Job drawing, mm, ordinate dimensions from the low corner. One solid piece. A direction names the side the tool comes from. Give positions to 0.01 mm unless a question says otherwise; leave off trailing zeros. Write each loop counter-clockwise with the first axis right and the second up, starting at its lowest first coordinate (ties: lowest second). Pieces come first, ordered by that corner, then holes. Notation, with made-up numbers: (15.5, 70) - (36.5, 70) arc R13 cw to (36.5, 89) - close; hole circle Ø7 at (6, -18). An arc over 180 degrees is marked (long way). Use a Markdown table: item, result. Add a question column.
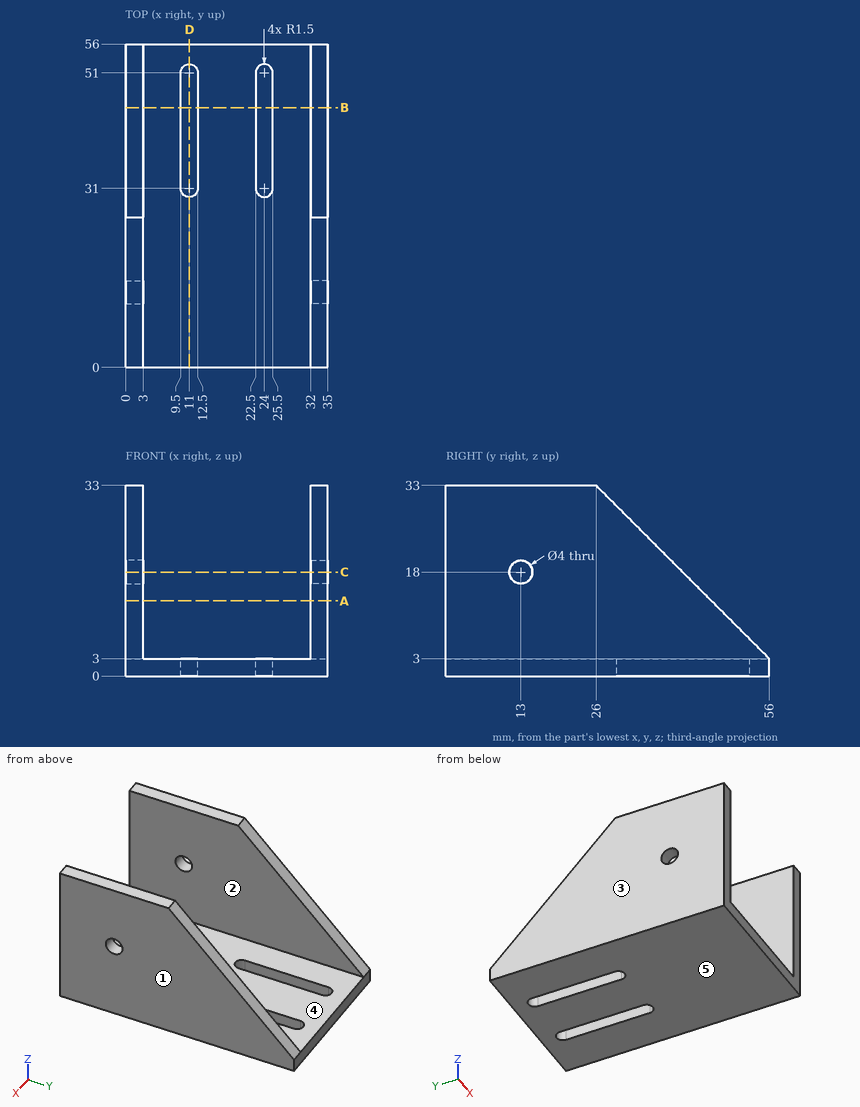
(1) Band-saw the part on C-C (z = 18). Write the cut outline in (x, y).
(2) Which spindle directions (+Z, -Z, +X, -X, +Y, -Y) get a long thin tool onto all of the face, cutting with end or side? Do the marked faces 4 and 5. Say none if no direction does.
(3) Band-saw the part on D-D (x = 11). Write the cut outline in (y, z).
(4) Flat gauge pin, fed straight in: pin 1 (12 mm diameter, centred on x = 27, z = 16, fed in from +Y). Where does the tip first touch, or does it go through?
(5) Two-plate mould, pull along X, no slides. Class the marked faces 1, 2 and 3: +X half, -X half, draft (parallel to the pull), parting line (faces both ways), or undercut.
(6) Band-saw the part on A-A (z = 13). Write the cut outline in (x, y), then the cut area to 3 significant figures.
(7) Band-saw the part on B-B (y = 45). Write the cut outline in (x, z), then the cut area to 3 significant figures.
(8) Probe probe 1 along X at (y, z) = (42, 2); probe 2 along Z at (x, y) = (1.65, 13); probe 3 along X at (y, z) = (27.5, 16.5). List the from-to ranges inside material, lowest first. Write a range as [from, to].
Model answer:
| question | item | result |
|---|---|---|
| 1 | outline | (0, 0) - (3, 0) - (3, 11) - (0, 11) - close; (0, 15) - (3, 15) - (3, 41) - (0, 41) - close; (32, 0) - (35, 0) - (35, 11) - (32, 11) - close; (32, 15) - (35, 15) - (35, 41) - (32, 41) - close |
| 2 | face 4 | +Z, +Y, -Y |
| 2 | face 5 | -Z, +X, -X, +Y, -Y |
| 3 | outline | (0, 0) - (29.5, 0) - (29.5, 3) - (0, 3) - close; (52.5, 0) - (56, 0) - (56, 3) - (52.5, 3) - close |
| 4 | pin 1 | stops at y = 46.32 |
| 5 | face 1 | +X half |
| 5 | face 2 | undercut |
| 5 | face 3 | -X half |
| 6 | outline | (0, 0) - (3, 0) - (3, 46) - (0, 46) - close; (32, 0) - (35, 0) - (35, 46) - (32, 46) - close |
| 6 | area | 276 mm^2 |
| 7 | outline | (0, 0) - (9.5, 0) - (9.5, 3) - (3, 3) - (3, 14) - (0, 14) - close; (12.5, 0) - (22.5, 0) - (22.5, 3) - (12.5, 3) - close; (25.5, 0) - (35, 0) - (35, 14) - (32, 14) - (32, 3) - (25.5, 3) - close |
| 7 | area | 153 mm^2 |
| 8 | probe 1 | x = [0, 9.5], [12.5, 22.5], [25.5, 35] |
| 8 | probe 2 | z = [0, 16], [20, 33] |
| 8 | probe 3 | x = [0, 3], [32, 35] |
